Autodesk Inventor part; units mm, degrees
ref_plane "YZ Plane" through (0, 0, 0) normal (1, 0, 0) x (0, 1, 0)
ref_plane "XZ Plane" through (0, 0, 0) normal (0, 1, 0) x (-1, 0, 0)
ref_plane "XY Plane" through (0, 0, 0) normal (0, 0, 1) x (1, 0, 0)
sketch "Sketch1" plane through (0, 0, 0) normal (0, 0, 1) x (1, 0, 0)
  circle A0 centre (0, 0) radius 50
  arc A1 (-2.5, 8.6458) -> (2.5, 8.6458) centre (0, 0) ccw
  line L0 (-2.5, 11.5) -> (2.5, 11.5)
  line L1 (2.5, 11.5) -> (2.5, 8.6458)
  line L2 (-2.5, 8.6458) -> (-2.5, 11.5)
  point P0 (0, 7.5)
  point P1 (0, 11.5)
  dimension "d0" = 100
  dimension "d1" = 18
  dimension "d3" = 5
  dimension "d4" = 0
  dimension "d5" = 11.5
extrude "Extrusion1" add sketch "Sketch1" along normal blind 3
equation "\"BendRadius\" = Thickness"
equation "\"BendReliefWidth\" = Thickness"
equation "\"BendReliefDepth\" = 0.5 * Thickness"
equation "\"CornerReliefSize\" = 4 * Thickness"
equation "\"MinimumRemnant\" = 2 * Thickness"
equation "\"TransitionRadius\" = BendRadius"
equation "\"JacobiRadiusSize\" = BendRadius"
equation "\"GapSize\" = Thickness"
properties part number "Brake disc"
Here's how the part is built. I have some questions about the finished solid (model axes, mm). A direction names the side the tool comes from. Round coordinates to 2 decimals unless told otherwise and drop trailing zeros. Loops run counter-clockwise (first coordinate to the right, second up) from the corner with the lowest first, then second, coordinate; pieces in that order, holes last. Notation, with made-up numbers: (-2.75, 68) - (14.25, 68) arc R36 ccw to (14.25, 104) - close; hole circle Ø1 at (13, 20). An arc over 180 degrees is marked (long way). One line per question, with ' | ' between items. Start each with the question number.
Q1. For faces 1 (the flat face through (2.5, 10, 1)), 2 (the flat face through (-1, -10, 3)), which set-ups out of +Z, -Z, +X, -X, +Y, -Y let a thin tool reach every point of the face, with its end or its side?
Q2. I want a section at C-C (z = 2). Write out the boundary of the cut face in (x, y).
Q3. I want a section at B-B (x = 0). Write out the boundary of the cut face in (y, z).
Q4. We'd pull the mould along X, two halves only. Please class faces 3 (the cylindrical face through (0, -9, 1)), 4 (the flat face through (-1, -10, 0)), 5 (the cylindrical face through (47.69, -15.02, 1.48)), 6 (the flat face through (0, 11.5, 1)): +X half, -X half, draft (parallel to the pull), parting line (faces both ways), or undercut.
Q5. Will these pins go through, and if not, where does the flat tip stop? pin 1 (1 mm diameter, centred on x = 25.5, z = 0.5, fed in from -Y); pin 2 (1 mm diameter, centred on x = -39.5, z = 2, fed in from -Y); pin 3 (0.9 mm diameter, centred on y = 10, z = 1.5, fed in from -X).
Q6. Please list where these lines run through material, in increasing order: line 1 (Y direction, x = 0, z = 1.6); line 2 (Y direction, x = 5, z = 2.6); line 3 (X direction, y = -42, z = 2). Write a range as [from, to].
Q7. I want a section at A-A (y = 0). Write out the boundary of the cut face in (x, z), then the cut area to 3 significant figures.
Q8. I want a section at D-D (y = -41). Write out the boundary of the cut face in (x, z).
Response values:
1) face 1: +Z, -Z | face 2: +Z, +X, -X, +Y, -Y
2) outline: circle Ø100 at (0, 0); hole (-2.5, 8.65) arc R9 ccw (long way) to (2.5, 8.65) - (2.5, 11.5) - (-2.5, 11.5) - close
3) outline: (-50, 0) - (-9, 0) - (-9, 3) - (-50, 3) - close; (11.5, 0) - (50, 0) - (50, 3) - (11.5, 3) - close
4) face 3: undercut | face 4: draft | face 5: parting line | face 6: undercut
5) pin 1: stops at y = -43.3 | pin 2: stops at y = -31.29 | pin 3: stops at x = -49.08
6) line 1: y = [-50, -9], [11.5, 50] | line 2: y = [-49.75, -7.48], [7.48, 49.75] | line 3: x = [-27.13, 27.13]
7) outline: (-50, 0) - (-9, 0) - (-9, 3) - (-50, 3) - close; (9, 0) - (50, 0) - (50, 3) - (9, 3) - close | area: 246 mm²
8) outline: (-28.62, 0) - (28.62, 0) - (28.62, 3) - (-28.62, 3) - close
